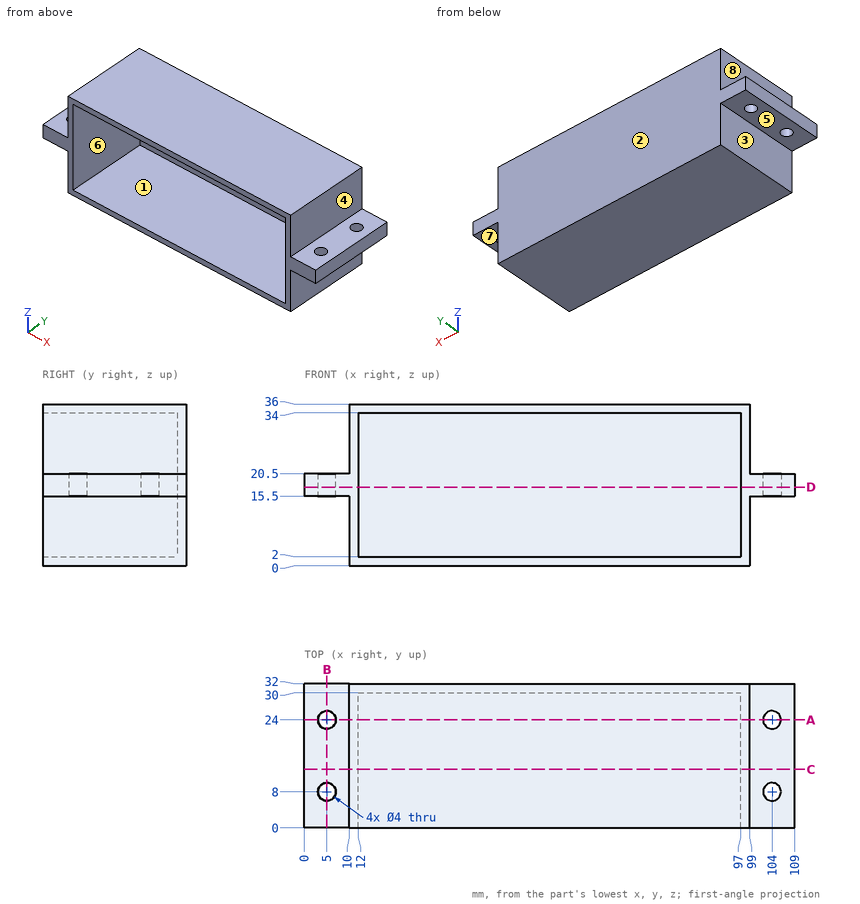
Could you check a few things on this drawing? It's one solid part, dimensions in mm from its lowest x, y, z. A direction names the side the tool comes from. Round coordinates to 2 decimals unless told otherwise and drop trailing zeros. Order: outer loops, then holes, each group sorted by start corner. A loop starts at its lowest first (then second) coordinate and runs counter-clockwise, first axis right, second up. Notation, with made-up numbers: M 3,-21 L 16,-21 A31 ccw 16,3 Z; hole C 13,11 d7. An arc over 180 degrees is marked long. Use a Markdown table: item, result.
1) If I drill on line 1 along Y through (x, z) = (5, 18); line 2 along X through (y, z) = (15, 5); line 3 along Z through (x, y) = (54, 18.5), over which ranges is the centre line in solid material (lowest first)?
Geometry says:
| item | result |
|---|---|
| line 1 | y = 0 to 6, 10 to 22, 26 to 32 |
| line 2 | x = 10 to 12, 97 to 99 |
| line 3 | z = 0 to 2, 34 to 36 |
2) If we mould it in two halves opening along X, with no side actions, what happens to the marked faces 1, 2 and 3? For each: +X half, -X half, draft (parallel to the pull), parting line (faces both ways), or undercut.
Geometry says:
| item | result |
|---|---|
| face 1 | undercut |
| face 2 | draft |
| face 3 | -X half |
3) Imagine slicing it at A-A (y = 24). List the corners of the cut face in (x, z) for me.
Geometry says:
| item | result |
|---|---|
| outline | M 0,15.5 L 3,15.5 L 3,20.5 L 0,20.5 Z; M 7,15.5 L 10,15.5 L 10,0 L 99,0 L 99,15.5 L 102,15.5 L 102,20.5 L 99,20.5 L 99,36 L 10,36 L 10,20.5 L 7,20.5 Z; M 106,15.5 L 109,15.5 L 109,20.5 L 106,20.5 Z; hole M 12,2 L 97,2 L 97,34 L 12,34 Z |
4) Imagine slicing it at C-C (y = 13). List the corners of the cut face in (x, z) for me.
Geometry says:
| item | result |
|---|---|
| outline | M 0,15.5 L 10,15.5 L 10,0 L 99,0 L 99,15.5 L 109,15.5 L 109,20.5 L 99,20.5 L 99,36 L 10,36 L 10,20.5 L 0,20.5 Z; hole M 12,2 L 97,2 L 97,34 L 12,34 Z |
5) On a 3-axis mill with a long thin cutter (end or side, diameter ignored), from which of +Z, -Z, +X, -X, +Y, -Y can I reach the whole of each face in a straight line? I mean the marked faces 4, 5, 6, 7 and 8. Say none if no direction works.
Geometry says:
| item | result |
|---|---|
| face 4 | +Z, +X, +Y, -Y |
| face 5 | -Z, -X, +Y, -Y |
| face 6 | -Y |
| face 7 | -Z, +X, +Y, -Y |
| face 8 | +Z, -X, +Y, -Y |
6) I'm going to push flat-ended pins straight in: P1, Ø3, axis at x = 104.5, y = 12, coming from the +Z side; P2, Ø3.5, axis at x = 5, y = 8, coming from the +Z side; P3, Ø4.5, axis at y = 17.5, z = 10.5, coming from the +X side; P4, Ø4.5, axis at x = 104, y = 24, coming from the -Z side. Where does each tip first touch, or does it pass through?
Geometry says:
| item | result |
|---|---|
| P1 | stops at z = 20.5 |
| P2 | passes through |
| P3 | stops at x = 99 |
| P4 | stops at z = 15.5 |
7) Imagine slicing it at D-D (z = 17.5). List the corners of the cut face in (x, y) for me, then the cut area to 3 significant figures.
Geometry says:
| item | result |
|---|---|
| outline | M 0,0 L 12,0 L 12,30 L 97,30 L 97,0 L 109,0 L 109,32 L 0,32 Z; hole C 5,8 d4; hole C 5,24 d4; hole C 104,8 d4; hole C 104,24 d4 |
| area | 888 mm² |
8) Imagine slicing it at B-B (x = 5). List the corners of the cut face in (y, z) for me.
Geometry says:
| item | result |
|---|---|
| outline | M 0,15.5 L 6,15.5 L 6,20.5 L 0,20.5 Z; M 10,15.5 L 22,15.5 L 22,20.5 L 10,20.5 Z; M 26,15.5 L 32,15.5 L 32,20.5 L 26,20.5 Z |
